Build history of the part. All positions in model axes, mm. Face numbers are marked on the shaded views. A direction names the side the tool comes from. Give positions to 0.01 mm unless a question says otherwise; leave off trailing zeros. Loops run counter-clockwise (first coordinate to the right, second up) from the corner with the lowest first, then second, coordinate; pieces in that order, holes last. Notation, with made-up numbers: M 28,28.25 L 39,28.25 A25 cw 39,40.25 Z; hole C -13.5,-19.75 d1. An arc over 180 degrees is marked long. Answer as a JSON object with one key per item and string values. Group by question number.
1. Drill centre lines: line 1 along Y through (x, z) = (2.9, -1.5); line 2 along Z through (x, y) = (2, 0.5); line 3 along Z through (x, y) = (0.35, -1.75). Where is each one in solid material? Low to high. Write a range as [from, to].
2. Slice it at A-A (z = 8.5). List the corners of the cut face in (x, y), then the cut area to 3 significant figures.
3. Slice it at B-B (x = 2). List the corners of the cut face in (y, z), then the cut area to 3 significant figures.
4. Drop a flat-ended pin along its axis: pin 1 Ø2 at (x, z) = (1.5, -1) entering from +Y. Give the stop position or say it passes through.
5. 3-axis set-ups, long thin cutter, end or side, ignore diameter. For the marked faces 1, 2 and 3: which of +Z, -Z, +X, -X, +Y, -Y reach the whole face in a straight line?
6. Slice it at C-C (z = 4). List the corners of the cut face in (x, y), then the cut area to 3 significant figures.
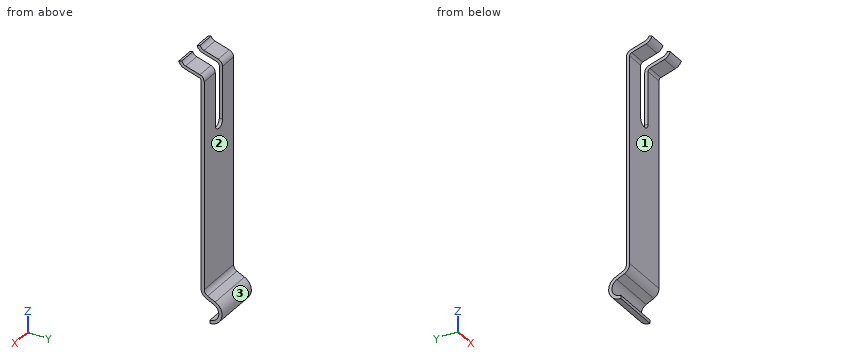
from build123d import *

# Parameters (mm, degrees)
BOSS_EXTRUDE1_DEPTH = 4
CUT_EXTRUDE1_DEPTH  = 4.15


with BuildPart() as part:
    # Sketch1 → Boss-Extrude1 (new body)
    with BuildSketch(Plane(origin=(0, 0, 0), x_dir=(0, 0, -1), z_dir=(1, 0, 0))):
        with BuildLine():
            Line((-9.035192226, 0), (8.097860886, 0))
            ThreePointArc((8.097860886, 0), (8.363999261, 0.076714795), (8.548470634, 0.283318539))
            Line((8.548470634, 0.283318539), (8.84623237, 0.902542447))
            ThreePointArc((8.84623237, 0.902542447), (9.969691043, 1.444171704), (10.747451865, 0.469179525))
            Line((10.747451865, 0.469179525), (10.477451865, 0.469179525))
            ThreePointArc((10.477451865, 0.469179525), (9.909686465, 1.180923816), (9.089561634, 0.785534458))
            Line((9.089561634, 0.785534458), (8.791799897, 0.166310551))
            ThreePointArc((8.791799897, 0.166310551), (8.507713984, -0.151859216), (8.097860886, -0.27))
            Line((8.097860886, -0.27), (-9.035192226, -0.27))
            ThreePointArc((-9.035192226, -0.27), (-9.172148547, -0.315221846), (-9.255249062, -0.433104643))
            Line((-9.255249062, -0.433104643), (-9.613802226, -1.612589711))
            ThreePointArc((-9.613802226, -1.612589711), (-9.79321671, -1.919973115), (-10.091698781, -2.113835356))
            Line((-10.091698781, -2.113835356), (-10.182452255, -1.859544564))
            ThreePointArc((-10.182452255, -1.859544564), (-9.988632728, -1.733659992), (-9.872129816, -1.534060379))
            Line((-9.872129816, -1.534060379), (-9.513576653, -0.354575311))
            ThreePointArc((-9.513576653, -0.354575311), (-9.332923359, -0.098308362), (-9.035192226, 0))
        make_face()
    extrude(amount=BOSS_EXTRUDE1_DEPTH)

    # Sketch2 → Cut-Extrude1 (cut)
    with BuildSketch(Plane(origin=(0, 0, 0), x_dir=(1, 0, 0), z_dir=(0, 1, 0))):
        with BuildLine():
            Line((1.5, -4.682452255), (1.5, -10.182452255))
            Line((1.5, -10.182452255), (2.5, -10.182452255))
            Line((2.5, -10.182452255), (2.5, -4.682452255))
            ThreePointArc((2.5, -4.682452255), (2, -4.182452255), (1.5, -4.682452255))
        make_face()
    extrude(amount=-CUT_EXTRUDE1_DEPTH, mode=Mode.SUBTRACT)


solid = part.part
Established:
{
 "1": {"line 1": "y = [-0.27, 0]", "line 2": "z = [-10.75, -10.48], [-8.95, -8.65]", "line 3": "z = [9.67, 10]"},
 "2": {"outline": "M 0,-0.27 L 1.5,-0.27 L 1.5,0 L 0,0 Z; M 2.5,-0.27 L 4,-0.27 L 4,0 L 2.5,0 Z", "area": "0.810 mm^2"},
 "3": {"outline": "M -0.27,-8.1 A0.77 ccw 0.17,-8.79 L 0.79,-9.09 A0.73 cw 0.47,-10.48 L 0.47,-10.75 A1 ccw 0.9,-8.85 L 0.28,-8.55 A0.5 cw 0,-8.1 L 0,4.18 L -0.27,4.18 Z", "area": "4.32 mm^2"},
 "4": {"pin 1": "stops at y = 0"},
 "5": {"face 1": "-Z, +X, -X, -Y", "face 2": "+Z, +X, -X, +Y", "face 3": "+X, -X, +Y"},
 "6": {"outline": "M 0,-0.27 L 4,-0.27 L 4,0 L 0,0 Z", "area": "1.08 mm^2"}
}
